Design review of the part built by this model. Coordinates are the model's own, in mm. A direction names the side the tool comes from. Give positions to 0.01 mm unless a question says otherwise; leave off trailing zeros. Loops run counter-clockwise (first coordinate to the right, second up) from the corner with the lowest first, then second, coordinate; pieces in that order, holes last. Notation, with made-up numbers: (6, 0.5) -> (30, 0.5) arc R16 ccw to (30, 17.5) -> close; hole circle Ø10 at (-5, -39). An arc over 180 degrees is marked (long way). Use a Markdown table: item, result. Add a question column.
1. For pin 1 Ø3.5 at (x, y) = (0, 0) entering from +Z (3 decimals); pin 2 Ø1.5 at (x, y) = (-2.5, -0.5) entering from +Z, all flat-tipped, find the tip position at first contact; note any pin that passes through.
2. Add section B-B (x = 0). State the section outline as (y, z) points (3 decimals), and give its area (3 significant figures).
3. Add section A-A (z = 6.25). State the section outline as (x, y) points.
4. To check wall thickness, follow line 1 (Y direction, x = -3.5, z = 5.25); line 2 (Y direction, x = 0, z = 2.5) (3 decimals). State the ranges of each line that lie inside material, in increasing order.
5. For faces 4 (the flat face through (0, -7, 8)), 5 (the flat face through (0, -6.25, 6)), list the 3-axis set-ups (+Z, -Z, +X, -X, +Y, -Y) from which the entire face can be reached by the end or side of a thin tool; tool diameter is ignored.
6. Draft analysis for pull direction X (two halves, no side actions). For faces 1 (the flat face through (7.5, 0, 3)), 2 (the flat face through (-2, 1, 5)), 3 (the cylindrical face through (1.34, -0.3, 2.53)), state which applies: pulls with the +X half, pulls with the -X half, needs draft (parallel to the pull), parting line crosses it, or undercut.
7. Add section C-C (y = 0). State the section outline as (x, z) points (3 decimals), and give its area (3 significant figures).
8. Add section D-D (z = 1). State the section outline as (x, y) points (3 decimals).
Solid Edge part; units mm, degrees
sketch "Sketch1" plane through (0, 0, 0) normal (1, 0, 0) x (0, 1, 0)
  line L0 (-7.5, 8) -> (-7.5, 0)
  line L1 (-7.5, 0) -> (7.5, 0)
  line L2 (7.5, 0) -> (7.5, 8)
  line L3 (7.5, 8) -> (6.25, 8)
  line L4 (6.25, 8) -> (6.25, 5)
  line L5 (6.25, 5) -> (-6.25, 5)
  line L6 (-6.25, 5) -> (-6.25, 8)
  line L7 (-6.25, 8) -> (-7.5, 8)
  dimension "D1" = 6.25
  dimension "D2" = 7.5
  dimension "D3" = 7.5
  dimension "D4" = 6.25
extrude "Protrusion1" add sketch "Sketch1" along normal mid plane 15
hole "screw_hole" at (0, 0, 0) direction (0, 0, 1) diameter 2.75 depth 30 tip angle 118 start chamfer 0.6 start chamfer angle 45 end chamfer 0.6 end chamfer angle 45
properties material "Polyethylene, low density"
Taken from the geometry:
| question | item | result |
|---|---|---|
| 1 | pin 1 | stops at z = 4.775 |
| 1 | pin 2 | stops at z = 5 |
| 2 | outline | (-7.5, 0) -> (-1.975, 0) -> (-1.375, 0.6) -> (-1.375, 4.4) -> (-1.975, 5) -> (-6.25, 5) -> (-6.25, 8) -> (-7.5, 8) -> close; (1.375, 0.6) -> (1.975, 0) -> (7.5, 0) -> (7.5, 8) -> (6.25, 8) -> (6.25, 5) -> (1.975, 5) -> (1.375, 4.4) -> close |
| 2 | area | 68.0 mm^2 |
| 3 | outline | (-7.5, -7.5) -> (7.5, -7.5) -> (7.5, -6.25) -> (-7.5, -6.25) -> close; (-7.5, 6.25) -> (7.5, 6.25) -> (7.5, 7.5) -> (-7.5, 7.5) -> close |
| 4 | line 1 | y = -7.5 to -6.25, 6.25 to 7.5 |
| 4 | line 2 | y = -7.5 to -1.375, 1.375 to 7.5 |
| 5 | face 4 | +Z, +X, -X, +Y, -Y |
| 5 | face 5 | +Z, +X, -X |
| 6 | face 1 | pulls with the +X half |
| 6 | face 2 | needs draft |
| 6 | face 3 | undercut |
| 7 | outline | (-7.5, 0) -> (-1.975, 0) -> (-1.375, 0.6) -> (-1.375, 4.4) -> (-1.975, 5) -> (-7.5, 5) -> close; (1.375, 0.6) -> (1.975, 0) -> (7.5, 0) -> (7.5, 5) -> (1.975, 5) -> (1.375, 4.4) -> close |
| 7 | area | 60.5 mm^2 |
| 8 | outline | (-7.5, -7.5) -> (7.5, -7.5) -> (7.5, 7.5) -> (-7.5, 7.5) -> close; hole circle Ø2.75 at (0, 0) |
